Answer from the drawing. Dimensions are ordinates in mm from the lowest x, y and z of the part. A direction names the side the tool comes from. Give positions to 0.01 mm unless a question says otherwise; leave off trailing zeros. Loops run counter-clockwise (first coordinate to the right, second up) from the corner with the lowest first, then second, coordinate; pieces in that order, holes last. Notation, with made-up numbers: M 74,-22.5 L 104,-22.5 A29 ccw 104,3.5 Z; hole C -0.5,-29.75 d5. An arc over 180 degrees is marked long. Use a Markdown table: item, result.
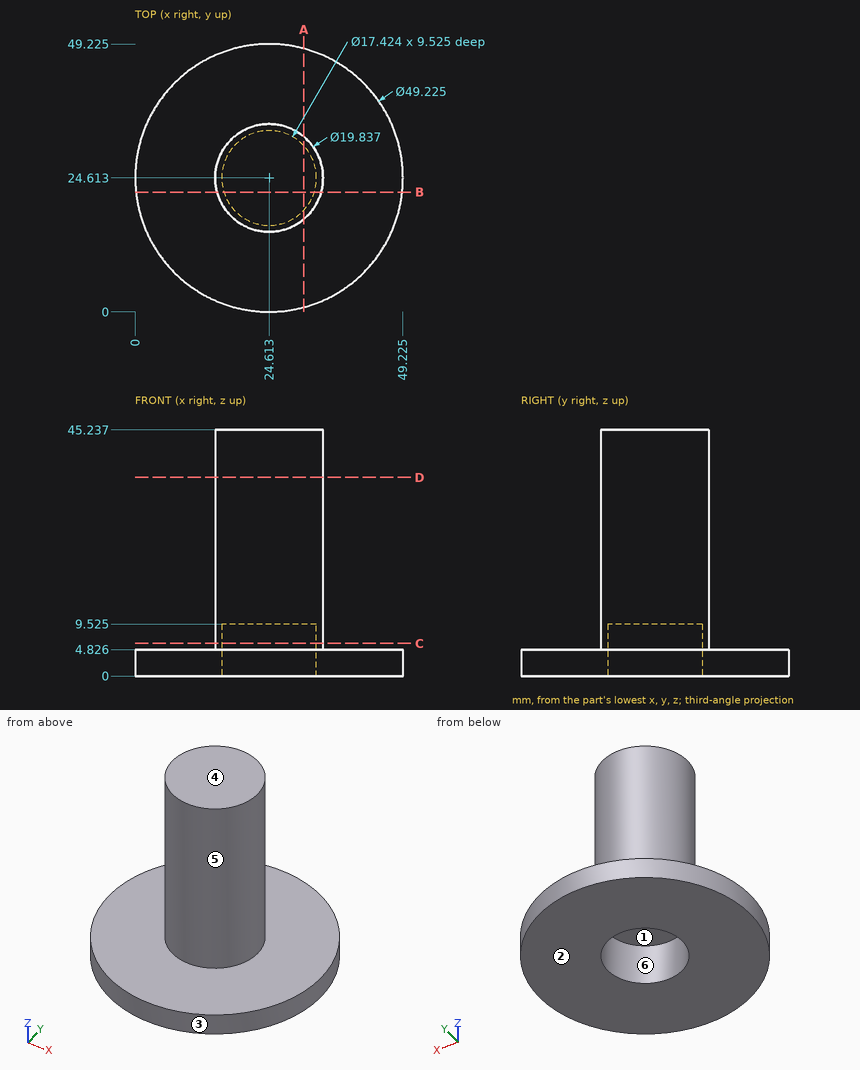
(1) Consider probe 1 along Z at (x, y) = (10, 12); probe 2 along Z at (x, y) = (27, 26) (1 decimal); probe 3 along Y at (x, z) = (19.5, 4.5) (1 decimal). Determine where each line is inside the solid, lowest interval first. Write a range as [from, to].
Entries:
| item | result |
|---|---|
| probe 1 | z = [0, 4.83] |
| probe 2 | z = [9.5, 45.2] |
| probe 3 | y = [0.5, 17.6], [31.7, 48.7] |
(2) A cutting plane is placed at B-B (y = 22). Write down the section's boundary in (x, z) (1 decimal), and give its area (3 significant figures).
Entries:
| item | result |
|---|---|
| outline | M 0.1,0 L 16.3,0 L 16.3,9.5 L 32.9,9.5 L 32.9,0 L 49.1,0 L 49.1,4.8 L 34.2,4.8 L 34.2,45.2 L 15,45.2 L 15,4.8 L 0.1,4.8 Z |
| area | 851 mm² |
(3) Which of the six approach directions +Z, -Z, +X, -X, +Y, -Y give full straight-line access (tool end or side, diameter ignored) to the marked faces 4, 5 and 6?
Entries:
| item | result |
|---|---|
| face 4 | +Z, +X, -X, +Y, -Y |
| face 5 | +Z |
| face 6 | -Z |
(4) A cutting plane is placed at D-D (z = 36.5). Write down the section's boundary in (x, y), and give its area (3 significant figures).
Entries:
| item | result |
|---|---|
| outline | C 24.61,24.61 d19.84 |
| area | 309 mm² |
(5) The mould has two halves that part along Y. Classify the marked faces 1, 2 and 3: released by +Y, released by -Y, zero draft, split by the parting line, or undercut.
Entries:
| item | result |
|---|---|
| face 1 | undercut |
| face 2 | zero draft |
| face 3 | split by the parting line |
(6) Given P1, Ø3, axis at y = 11.5, z = 37, coming from the +X side; P2, Ø10, axis at x = 21, z = 15.5, coming from the +Y side; P3, Ø14, axis at x = 25.5, y = 23.5, coming from the -Z side (3 decimals); P4, Ø2, axis at y = 28, z = 21, coming from the +X side, each flat-ended and moving along its own axis, determine where each tip first touches the part or whether it passes through.
Entries:
| item | result |
|---|---|
| P1 | passes through |
| P2 | stops at y = 34.53 |
| P3 | stops at z = 9.525 |
| P4 | stops at x = 34.24 |
(7) A cutting plane is placed at A-A (x = 31). Write down the section's boundary in (y, z) (1 decimal).
Entries:
| item | result |
|---|---|
| outline | M 0.8,0 L 18.7,0 L 18.7,9.5 L 30.5,9.5 L 30.5,0 L 48.4,0 L 48.4,4.8 L 32.2,4.8 L 32.2,45.2 L 17,45.2 L 17,4.8 L 0.8,4.8 Z |
(8) A cutting plane is placed at C-C (z = 6). Write down the section's boundary in (x, y) (1 decimal).
Entries:
| item | result |
|---|---|
| outline | C 24.6,24.6 d19.8; hole C 24.6,24.6 d17.4 |
